from build123d import *

# Parameters (mm, degrees)
SKETCH1_R           = 2.5
SKETCH1_R_2         = 6
BOSS_EXTRUDE1_DEPTH = 1964


with BuildPart() as part:
    # Sketch1 → Boss-Extrude1 (new body)
    with BuildSketch(Plane.XY):
        with BuildLine():
            Line((-17, -40), (-4.1, -40))
            Line((-4.1, -40), (-4.1, -37))
            Line((-4.1, -37), (-10.5, -37))
            Line((-10.5, -37), (-10.5, -33.6627417))
            ThreePointArc((-10.5, -33.6627417), (-10.378207252, -33.050448208), (-10.03137085, -32.53137085))
            Line((-10.03137085, -32.53137085), (-7.464466094, -29.964466094))
            ThreePointArc((-7.464466094, -29.964466094), (-5.84234935, -28.880602337), (-3.928932188, -28.5))
            Line((-3.928932188, -28.5), (3.928932188, -28.5))
            ThreePointArc((3.928932188, -28.5), (5.84234935, -28.880602337), (7.464466094, -29.964466094))
            Line((7.464466094, -29.964466094), (10.03137085, -32.53137085))
            ThreePointArc((10.03137085, -32.53137085), (10.378207252, -33.050448208), (10.5, -33.6627417))
            Line((10.5, -33.6627417), (10.5, -37))
            Line((10.5, -37), (4.1, -37))
            Line((4.1, -37), (4.1, -40))
            Line((4.1, -40), (17, -40))
            ThreePointArc((17, -40), (19.121320344, -39.121320344), (20, -37))
            Line((20, -37), (20, -24.1))
            Line((20, -24.1), (17, -24.1))
            Line((17, -24.1), (17, -30.5))
            Line((17, -30.5), (13.6627417, -30.5))
            ThreePointArc((13.6627417, -30.5), (13.050448208, -30.378207252), (12.53137085, -30.03137085))
            Line((12.53137085, -30.03137085), (9.964466094, -27.464466094))
            ThreePointArc((9.964466094, -27.464466094), (8.880602337, -25.84234935), (8.5, -23.928932188))
            Line((8.5, -23.928932188), (8.5, -16.071067812))
            ThreePointArc((8.5, -16.071067812), (8.880602337, -14.15765065), (9.964466094, -12.535533906))
            Line((9.964466094, -12.535533906), (12.53137085, -9.96862915))
            ThreePointArc((12.53137085, -9.96862915), (13.050448208, -9.621792748), (13.6627417, -9.5))
            Line((13.6627417, -9.5), (17, -9.5))
            Line((17, -9.5), (17, -15.9))
            Line((17, -15.9), (20, -15.9))
            Line((20, -15.9), (20, 15.9))
            Line((20, 15.9), (17, 15.9))
            Line((17, 15.9), (17, 9.5))
            Line((17, 9.5), (13.6627417, 9.5))
            ThreePointArc((13.6627417, 9.5), (13.050448208, 9.621792748), (12.53137085, 9.96862915))
            Line((12.53137085, 9.96862915), (9.964466094, 12.535533906))
            ThreePointArc((9.964466094, 12.535533906), (8.880602337, 14.15765065), (8.5, 16.071067812))
            Line((8.5, 16.071067812), (8.5, 23.928932188))
            ThreePointArc((8.5, 23.928932188), (8.880602337, 25.84234935), (9.964466094, 27.464466094))
            Line((9.964466094, 27.464466094), (12.53137085, 30.03137085))
            ThreePointArc((12.53137085, 30.03137085), (13.050448208, 30.378207252), (13.6627417, 30.5))
            Line((13.6627417, 30.5), (17, 30.5))
            Line((17, 30.5), (17, 24.1))
            Line((17, 24.1), (20, 24.1))
            Line((20, 24.1), (20, 37))
            ThreePointArc((20, 37), (19.121320344, 39.121320344), (17, 40))
            Line((17, 40), (4.1, 40))
            Line((4.1, 40), (4.1, 37))
            Line((4.1, 37), (10.5, 37))
            Line((10.5, 37), (10.5, 33.6627417))
            ThreePointArc((10.5, 33.6627417), (10.378207252, 33.050448208), (10.03137085, 32.53137085))
            Line((10.03137085, 32.53137085), (7.464466094, 29.964466094))
            ThreePointArc((7.464466094, 29.964466094), (5.84234935, 28.880602337), (3.928932188, 28.5))
            Line((3.928932188, 28.5), (-3.928932188, 28.5))
            ThreePointArc((-3.928932188, 28.5), (-5.84234935, 28.880602337), (-7.464466094, 29.964466094))
            Line((-7.464466094, 29.964466094), (-10.03137085, 32.53137085))
            ThreePointArc((-10.03137085, 32.53137085), (-10.378207252, 33.050448208), (-10.5, 33.6627417))
            Line((-10.5, 33.6627417), (-10.5, 37))
            Line((-10.5, 37), (-4.1, 37))
            Line((-4.1, 37), (-4.1, 40))
            Line((-4.1, 40), (-17, 40))
            ThreePointArc((-17, 40), (-19.121320344, 39.121320344), (-20, 37))
            Line((-20, 37), (-20, 24.1))
            Line((-20, 24.1), (-17, 24.1))
            Line((-17, 24.1), (-17, 30.5))
            Line((-17, 30.5), (-13.6627417, 30.5))
            ThreePointArc((-13.6627417, 30.5), (-13.050448208, 30.378207252), (-12.53137085, 30.03137085))
            Line((-12.53137085, 30.03137085), (-9.964466094, 27.464466094))
            ThreePointArc((-9.964466094, 27.464466094), (-8.880602337, 25.84234935), (-8.5, 23.928932188))
            Line((-8.5, 23.928932188), (-8.5, 16.071067812))
            ThreePointArc((-8.5, 16.071067812), (-8.880602337, 14.15765065), (-9.964466094, 12.535533906))
            Line((-9.964466094, 12.535533906), (-12.53137085, 9.96862915))
            ThreePointArc((-12.53137085, 9.96862915), (-13.050448208, 9.621792748), (-13.6627417, 9.5))
            Line((-13.6627417, 9.5), (-17, 9.5))
            Line((-17, 9.5), (-17, 15.9))
            Line((-17, 15.9), (-20, 15.9))
            Line((-20, 15.9), (-20, -15.9))
            Line((-20, -15.9), (-17, -15.9))
            Line((-17, -15.9), (-17, -9.5))
            Line((-17, -9.5), (-13.6627417, -9.5))
            ThreePointArc((-13.6627417, -9.5), (-13.050448208, -9.621792748), (-12.53137085, -9.96862915))
            Line((-12.53137085, -9.96862915), (-9.964466094, -12.535533906))
            ThreePointArc((-9.964466094, -12.535533906), (-8.880602337, -14.15765065), (-8.5, -16.071067812))
            Line((-8.5, -16.071067812), (-8.5, -23.928932188))
            ThreePointArc((-8.5, -23.928932188), (-8.880602337, -25.84234935), (-9.964466094, -27.464466094))
            Line((-9.964466094, -27.464466094), (-12.53137085, -30.03137085))
            ThreePointArc((-12.53137085, -30.03137085), (-13.050448208, -30.378207252), (-13.6627417, -30.5))
            Line((-13.6627417, -30.5), (-17, -30.5))
            Line((-17, -30.5), (-17, -24.1))
            Line((-17, -24.1), (-20, -24.1))
            Line((-20, -24.1), (-20, -37))
            ThreePointArc((-20, -37), (-19.121320344, -39.121320344), (-17, -40))
        make_face()
        with Locations((15, 35)):
            Circle(SKETCH1_R, mode=Mode.SUBTRACT)
        with Locations((15, -35)):
            Circle(SKETCH1_R, mode=Mode.SUBTRACT)
        with Locations((0, 20)):
            Circle(SKETCH1_R_2, mode=Mode.SUBTRACT)
        with Locations((0, -20)):
            Circle(SKETCH1_R_2, mode=Mode.SUBTRACT)
        with Locations((-15, 35)):
            Circle(SKETCH1_R, mode=Mode.SUBTRACT)
        with Locations((-15, -35)):
            Circle(SKETCH1_R, mode=Mode.SUBTRACT)
        with BuildLine():
            Line((-14.242640687, -4.242640687), (-9.949747468, -8.535533906))
            ThreePointArc((-9.949747468, -8.535533906), (-8.327630724, -9.619397663), (-6.414213562, -10))
            Line((-6.414213562, -10), (6.414213562, -10))
            ThreePointArc((6.414213562, -10), (8.327630724, -9.619397663), (9.949747468, -8.535533906))
            Line((9.949747468, -8.535533906), (14.242640687, -4.242640687))
            ThreePointArc((14.242640687, -4.242640687), (16, 0), (14.242640687, 4.242640687))
            Line((14.242640687, 4.242640687), (9.949747468, 8.535533906))
            ThreePointArc((9.949747468, 8.535533906), (8.327630724, 9.619397663), (6.414213562, 10))
            Line((6.414213562, 10), (-6.414213562, 10))
            ThreePointArc((-6.414213562, 10), (-8.327630724, 9.619397663), (-9.949747468, 8.535533906))
            Line((-9.949747468, 8.535533906), (-14.242640687, 4.242640687))
            ThreePointArc((-14.242640687, 4.242640687), (-16, 0), (-14.242640687, -4.242640687))
        make_face(mode=Mode.SUBTRACT)
    extrude(amount=-BOSS_EXTRUDE1_DEPTH)


solid = part.part
Can you work these out from the model? Positions are in its coordinate system, mm. Coordinates: 2 decimals unless noted, no trailing zeros. Use one line per item in the form item = value.
Q1. For P1, Ø4, axis at y = 21.5, z = -606.5, coming from the -X side; P2, Ø2.5, axis at x = 18.5, z = -1322.5, coming from the -Y side, each with a flat end and sliding along its axis, tell me the tip position at first contact or that it passes through.
Model answer:
P1 = -8.5
P2 = -39.99
Q2. If we section it at A-A (z = -455): State how many separate pieces and enclosed holes the cut face has, then the cut area to 3 significant figures.
Model answer:
separate_pieces = 1
enclosed_holes = 7
area = 1,280 mm^2
Q3. I need wall thicknesses on line 1 along Y through (x, z) = (1, -1024.5); line 2 along X through (y, z) = (-15.5, -477.5); line 3 along Y through (x, z) = (-14, -536). Which ranges of each line are inside material? Lowest first, please. Write a range as from..to.
Model answer:
line_1 = -28.5..-25.92, -14.08..-10, 10..14.08, 25.92..28.5
line_2 = -20..-17, -8.53..-3.97, 3.97..8.53, 17..20
line_3 = -40..-37.29, -32.71..-30.5, -9.5..-4.49, 4.49..9.5, 30.5..32.71, 37.29..40
